from build123d import *

# Parameters (mm, degrees)
SKETCH1_W                      = 25
SKETCH1_H                      = 20
BOSS_EXTRUDE1_DEPTH            = 1.5
SKETCH2_W                      = 15
SKETCH2_H                      = 3
BOSS_EXTRUDE2_DEPTH            = 15
CUT_EXTRUDE1_REACH             = 20
SKETCH3_R                      = 2.1
CUT_EXTRUDE1_DIRECTION_2_DEPTH = 1


with BuildPart() as part:
    # Sketch1 → Boss-Extrude1 (new body, symmetric)
    with BuildSketch(Plane(origin=(0, 0, 0), x_dir=(1, 0, 0), z_dir=(0, 1, 0))):
        Rectangle(SKETCH1_W, SKETCH1_H)
    extrude(amount=BOSS_EXTRUDE1_DEPTH, both=True)

    # Sketch2 → Boss-Extrude2 (add)
    with BuildSketch(Plane.XZ.offset(1.5)):
        Rectangle(SKETCH2_W, SKETCH2_H)
    extrude(amount=BOSS_EXTRUDE2_DEPTH)

    # Sketch3 → Cut-Extrude1 (cut, up to next)
    with BuildSketch(Plane(origin=(0, 1.5, 0), x_dir=(1, 0, 0), z_dir=(0, 1, 0)), mode=Mode.PRIVATE) as cut_extrude1_sk1:
        with Locations((-8, 6)):
            Circle(SKETCH3_R)
    cut_extrude1_tool1 = extrude(cut_extrude1_sk1.sketch, amount=-CUT_EXTRUDE1_REACH, mode=Mode.PRIVATE) & part.part
    add(cut_extrude1_tool1.solids().sort_by_distance((-8, 1.5, -6))[0], mode=Mode.SUBTRACT)
    # Sketch3 → Cut-Extrude1 (cut, up to next)
    with BuildSketch(Plane(origin=(0, 1.5, 0), x_dir=(1, 0, 0), z_dir=(0, 1, 0)), mode=Mode.PRIVATE) as cut_extrude1_sk2:
        with Locations((8, 6)):
            Circle(SKETCH3_R)
    cut_extrude1_tool2 = extrude(cut_extrude1_sk2.sketch, amount=-CUT_EXTRUDE1_REACH, mode=Mode.PRIVATE) & part.part
    add(cut_extrude1_tool2.solids().sort_by_distance((8, 1.5, -6))[0], mode=Mode.SUBTRACT)
    # Sketch3 → Cut-Extrude1 (cut, up to next)
    with BuildSketch(Plane(origin=(0, 1.5, 0), x_dir=(1, 0, 0), z_dir=(0, 1, 0)), mode=Mode.PRIVATE) as cut_extrude1_sk3:
        with Locations((8, -6)):
            Circle(SKETCH3_R)
    cut_extrude1_tool3 = extrude(cut_extrude1_sk3.sketch, amount=-CUT_EXTRUDE1_REACH, mode=Mode.PRIVATE) & part.part
    add(cut_extrude1_tool3.solids().sort_by_distance((8, 1.5, 6))[0], mode=Mode.SUBTRACT)
    # Sketch3 → Cut-Extrude1 (cut, up to next)
    with BuildSketch(Plane(origin=(0, 1.5, 0), x_dir=(1, 0, 0), z_dir=(0, 1, 0)), mode=Mode.PRIVATE) as cut_extrude1_sk4:
        with Locations((-8, -6)):
            Circle(SKETCH3_R)
    cut_extrude1_tool4 = extrude(cut_extrude1_sk4.sketch, amount=-CUT_EXTRUDE1_REACH, mode=Mode.PRIVATE) & part.part
    add(cut_extrude1_tool4.solids().sort_by_distance((-8, 1.5, 6))[0], mode=Mode.SUBTRACT)

    # Sketch3 → Cut-Extrude1 direction 2 (cut)
    with BuildSketch(Plane(origin=(0, 1.5, 0), x_dir=(1, 0, 0), z_dir=(0, 1, 0))):
        with Locations((-8, 6)):
            Circle(SKETCH3_R)
        with Locations((8, 6)):
            Circle(SKETCH3_R)
        with Locations((8, -6)):
            Circle(SKETCH3_R)
        with Locations((-8, -6)):
            Circle(SKETCH3_R)
    extrude(amount=CUT_EXTRUDE1_DIRECTION_2_DEPTH, mode=Mode.SUBTRACT)


solid = part.part
Build history of the part. All positions in model axes, mm. A direction names the side the tool comes from. Round coordinates to 2 decimals unless told otherwise and drop trailing zeros. Write each loop counter-clockwise with the first axis right and the second up, starting at its lowest first coordinate (ties: lowest second). Pieces come first, ordered by that corner, then holes. Notation, with made-up numbers: M 80,-13 L 117,-13 A12 ccw 117,-7 Z; hole C 41.25,41 d10. An arc over 180 degrees is marked long. Answer as a JSON object with one key per item and string values. Group by question number.
(1) Drill centre lines: L1, parallel to Z at x = -8, y = -0.1; L2, parallel to X at y = 0.7, z = -6; L3, parallel to Z at x = -6.75, y = -6.75. Where is each one in solid material? Low to high.
(2) Cut at A-A (z = -6). Give the cut face in (x, y), and give its area (3 significant figures).
(3) Flat gauge pins, fed straight in: pin 1 (1 mm diameter, centred on y = -13.5, z = -1, fed in from +X); pin 2 (1.5 mm diameter, centred on x = -4, z = -7, fed in from -Y); pin 3 (3.5 mm diameter, centred on x = 8, z = 6, fed in from +Y); pin 4 (1.5 mm diameter, centred on y = -10.5, z = 0.5, fed in from -X). Where does each tip first touch, or does it go through?
(4) Which spindle directions (+Z, -Z, +X, -X, +Y, -Y) get a long thin tool onto all of the face, cutting with end or side? Do faces 4 (the cylindrical face through (-10.1, 0.02, 5.91)), 5 (the flat face through (0, -9, -1.5)), 6 (the flat face through (-7.5, -9, 0)), 7 (the flat face through (-12.5, 0, 0)), 8 (the flat face through (7.5, -9, 0)). Say none if no direction does.
(5) Cut at C-C (y = -0.25). Give the cut face in (x, z), and give its area (3 significant figures).
(6) Cut at D-D (x = 1). Give the cut face in (y, z), and give its area (3 significant figures).
(7) Cut at B-B (x = 8). Give the cut face in (y, z).
(8) Mould opens along Z. For faces 1 (the flat face through (0, -16.5, 0)), 2 (the cylindrical face through (6.452, 0.021, -7.419)), 3 (the flat face through (0, -9, 1.5)) say: pulls with the +Z half, pulls with the -Z half, needs draft (parallel to the pull), parting line crosses it, or undercut.
Responses:
{
 "1": {"L1": "z = -10 to -8.1, -3.9 to 3.9, 8.1 to 10", "L2": "x = -12.5 to -10.1, -5.9 to 5.9, 10.1 to 12.5", "L3": "z = -1.5 to 1.5"},
 "2": {"outline": "M -12.5,-1.5 L -10.1,-1.5 L -10.1,1.5 L -12.5,1.5 Z; M -5.9,-1.5 L 5.9,-1.5 L 5.9,1.5 L -5.9,1.5 Z; M 10.1,-1.5 L 12.5,-1.5 L 12.5,1.5 L 10.1,1.5 Z", "area": "49.8 mm2"},
 "3": {"pin 1": "stops at x = 7.5", "pin 2": "stops at y = -1.5", "pin 3": "passes through", "pin 4": "stops at x = -7.5"},
 "4": {"face 4": "+Y, -Y", "face 5": "-Z, +X, -X, -Y", "face 6": "+Z, -Z, -X, -Y", "face 7": "+Z, -Z, -X, +Y, -Y", "face 8": "+Z, -Z, +X, -Y"},
 "5": {"outline": "M -12.5,-10 L 12.5,-10 L 12.5,10 L -12.5,10 Z; hole C -8,-6 d4.2; hole C -8,6 d4.2; hole C 8,-6 d4.2; hole C 8,6 d4.2", "area": "445 mm2"},
 "6": {"outline": "M -16.5,-1.5 L -1.5,-1.5 L -1.5,-10 L 1.5,-10 L 1.5,10 L -1.5,10 L -1.5,1.5 L -16.5,1.5 Z", "area": "105 mm2"},
 "7": {"outline": "M -1.5,-10 L 1.5,-10 L 1.5,-8.1 L -1.5,-8.1 Z; M -1.5,-3.9 L 1.5,-3.9 L 1.5,3.9 L -1.5,3.9 Z; M -1.5,8.1 L 1.5,8.1 L 1.5,10 L -1.5,10 Z"},
 "8": {"face 1": "needs draft", "face 2": "undercut", "face 3": "pulls with the +Z half"}
}
